Geometry: see drawing. Coordinates: mm, zero at the bounding-box minimum. A direction names the side the tool comes from. Give positions to 0.01 mm unless a question says otherwise; leave off trailing zeros. Loops run counter-clockwise (first coordinate to the right, second up) from the corner with the lowest first, then second, coordinate; pieces in that order, holes last. Notation, with made-up numbers: (19.25, 50) -> (24.25, 50) arc R32 cw to (24.25, 81) -> close; hole circle Ø3 at (16.25, 50). An arc over 180 degrees is marked (long way). One line per question, with ' | ' between items.
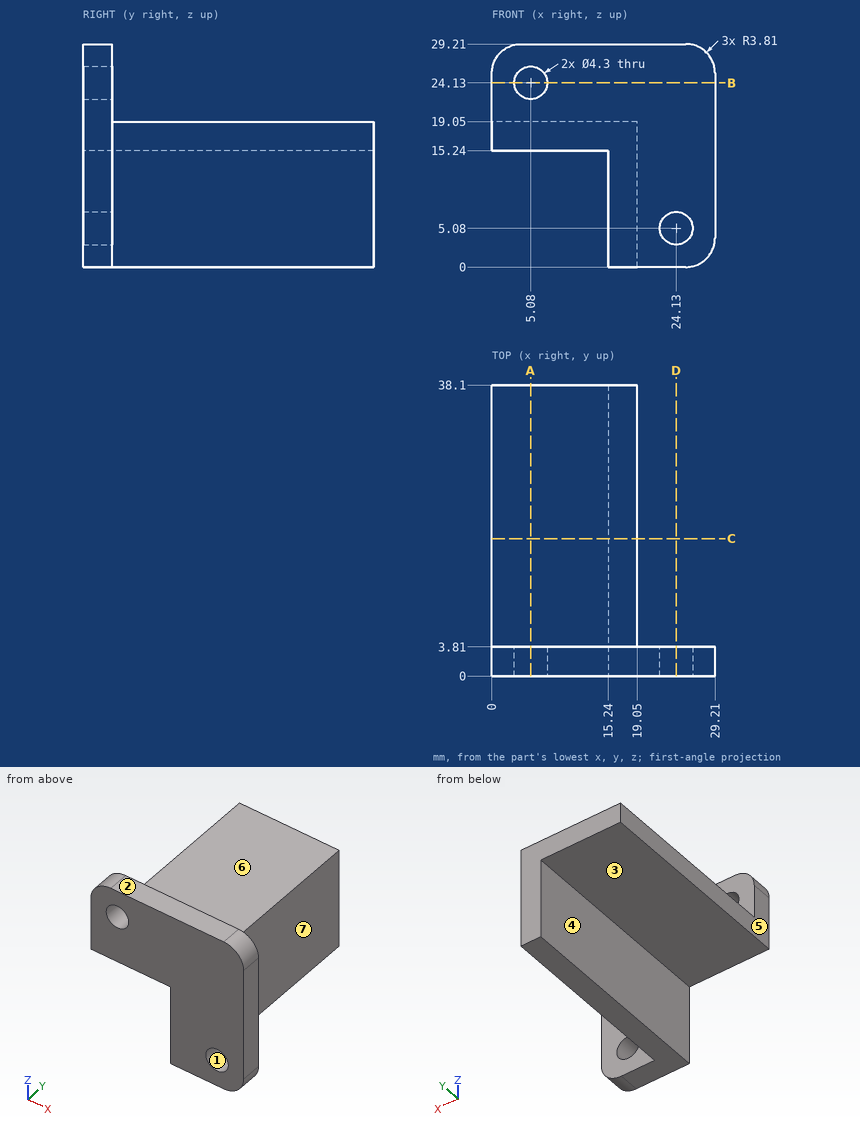
1. Section query B-B (z = 24.13). Output: boundary loops of the cut face in (x, y), then the cut area to 3 significant figures.
Determined:
outline: (0, 0) -> (2.93, 0) -> (2.93, 3.81) -> (0, 3.81) -> close; (7.23, 0) -> (29.21, 0) -> (29.21, 3.81) -> (7.23, 3.81) -> close | area: 94.9 mm2
2. Pull-direction query (Z, two-part tool) for the marked faces 1, 2 and 3; classes: pulls with the +Z half, pulls with the -Z half, needs draft (parallel to the pull), parting line crosses it, or undercut.
Determined:
face 1: undercut | face 2: pulls with the +Z half | face 3: pulls with the -Z half
3. Pin query (flat end, axial travel): P1, Ø4, axis at x = 12, y = 16, coming from the +Z side; P2, Ø15, axis at y = 14.5, z = 7.5, coming from the +X side; P3, Ø7, axis at x = 5.08, z = 24.13, coming from the +Y side. Return the tip coordinate at first contact, or that it passes through.
Determined:
P1: stops at z = 19.05 | P2: stops at x = 19.05 | P3: stops at y = 3.81
4. Section query A-A (x = 5.08). Output: boundary loops of the cut face in (y, z), then the cut area to 3 significant figures.
Determined:
outline: (0, 15.24) -> (38.1, 15.24) -> (38.1, 19.05) -> (3.81, 19.05) -> (3.81, 21.98) -> (0, 21.98) -> close; (0, 26.28) -> (3.81, 26.28) -> (3.81, 29.21) -> (0, 29.21) -> close | area: 167 mm2
5. Section query C-C (y = 18). Output: boundary loops of the cut face in (x, z), then the cut area to 3 significant figures.
Determined:
outline: (0, 15.24) -> (15.24, 15.24) -> (15.24, 0) -> (19.05, 0) -> (19.05, 19.05) -> (0, 19.05) -> close | area: 131 mm2
6. Ray query, line 1 along Z through (x, y) = (24.13, 1.95); line 2 along Z through (x, y) = (5.08, 2.75); line 3 along X through (y, z) = (17.5, 7). Return the intervals inside material, ascending. Write a range as from..to.
Determined:
line 1: z = 0..2.93, 7.23..29.21 | line 2: z = 15.24..21.98, 26.28..29.21 | line 3: x = 15.24..19.05
7. Section query D-D (x = 24.13). Output: boundary loops of the cut face in (y, z), then the cut area to 3 significant figures.
Determined:
outline: (0, 0) -> (3.81, 0) -> (3.81, 2.93) -> (0, 2.93) -> close; (0, 7.23) -> (3.81, 7.23) -> (3.81, 29.21) -> (0, 29.21) -> close | area: 94.9 mm2
8. Reachability of the marked faces 4, 5, 6 and 7 from +Z, -Z, +X, -X, +Y, -Y: full face, straight path, thin tool, end or side. Return the list, or none.
Determined:
face 4: -Z, -X, +Y, -Y | face 5: +Z, -Z, -X, +Y, -Y | face 6: +Z, +X, -X, +Y | face 7: +Z, -Z, +X, +Y
